Work out the finished part from the listing and answer in its coordinate system (mm). A direction names the side the tool comes from. Round coordinates to 2 decimals unless told otherwise and drop trailing zeros. Order: outer loops, then holes, each group sorted by start corner. A loop starts at its lowest first (then second) coordinate and runs counter-clockwise, first axis right, second up. Notation, with made-up numbers: (28.5, 32) - (43.5, 32) arc R20 cw to (43.5, 36) - close; hole circle Ø1 at (-8, 84.5). An arc over 180 degrees is marked (long way). Use one line per item in the form item = value. Start each with the question number.
Q1. The part is cut by section B-B on y = -13. Determine the outline of the cut face in (x, z), plus the area to 3 significant figures.
Q2. Which of the six approach directions +Z, -Z, +X, -X, +Y, -Y give full straight-line access (tool end or side, diameter ignored) to faces 1 (the flat face through (0, 9, 0)), 2 (the flat face through (-11, 11, 0)), 3 (the cylindrical face through (-1.172, -17.944, 8.923))?
Q3. The part is cut by section A-A on y = 6. Determine the outline of the cut face in (x, z), plus the area to 3 significant figures.
Q4. Find the intervals of material crossed by line 1 (Y direction, x = -14.5, z = -3.5); line 2 (Y direction, x = -5, z = 8); line 3 (X direction, y = -6, z = -11), in increasing order. Write a range as [from, to].
Q5. Given P1, Ø3.5, axis at y = 9.5, z = 0, coming from the +X side; P2, Ø8, axis at y = -8, z = -4.5, coming from the -X side; P3, Ø1, axis at x = 11.5, z = -7, coming from the +Y side; P4, Ø6, axis at y = -18.5, z = -10.5, coming from the -X side, each flat-ended and moving along its own axis, determine where each tip first touches the part or whether it passes through.
from build123d import *

# Parameters (mm, degrees)
F0_R          = 18
F1_DEPTH      = 7
F2_R          = 14
F3_DEPTH      = 14
F4_R          = 9
F5_DEPTH      = 23
F6_W          = 22
F6_H          = 3
F7_DEPTH      = 7
F7_DEPTH_BACK = 11
F8_SIZE       = 1
F9_SIZE       = 1


with BuildPart() as f1:
    # F0 (on Front) → F1 (new body, symmetric)
    with BuildSketch(Plane.XZ):
        Circle(F0_R)
    extrude(amount=F1_DEPTH, both=True)

    # F2 (on Front) → F3 (join)
    with BuildSketch(Plane.XZ):
        Circle(F2_R)
    extrude(amount=F3_DEPTH)

    # F4 (on Front) → F5 (join)
    with BuildSketch(Plane.XZ):
        Circle(F4_R)
    extrude(amount=F5_DEPTH)

    # F6 (on Front) → F7 (join, two sides)
    with BuildSketch(Plane.XZ) as f7_sk:
        with Locations((-11, 0)):
            Rectangle(F6_W, F6_H)
    extrude(amount=F7_DEPTH)
    extrude(f7_sk.sketch, amount=-F7_DEPTH_BACK)

    # F8
    f8_edges = [f1.edges().sort_by_distance(p)[0] for p in [
        (-9, -23, 0),
    ]]
    chamfer(f8_edges, length=F8_SIZE)

    # F9
    f9_edges = [f1.edges().sort_by_distance(p)[0] for p in [
        (0.750653, -7, -17.984341),
        (0.750653, -7, 17.984341),
    ]]
    chamfer(f9_edges, length=F9_SIZE)


solid = f1.part
Found:
q1.outline = circle Ø28 at (0, 0)
q1.area = 616 mm²
q2.face_1 = +Z, -Z, +X, +Y
q2.face_2 = +Z, -Z, +X, -X, +Y
q2.face_3 = -Y
q3.outline = (-22, -1.5) - (-17.94, -1.5) arc R18 ccw (long way) to (-17.94, 1.5) - (-22, 1.5) - close
q3.area = 1,030 mm²
q4.line_1 = [-7, 7]
q4.line_2 = [-14, 7]
q4.line_3 = [-14.25, 14.25]
q5.P1 = 0
q5.P2 = -22
q5.P3 = 7
q5.P4 = -4.97
